Autodesk Inventor part; units mm, degrees
ref_plane "YZ Plane" through (0, 0, 0) normal (1, 0, 0) x (0, 1, 0)
ref_plane "XZ Plane" through (0, 0, 0) normal (0, 1, 0) x (-1, 0, 0)
ref_plane "XY Plane" through (0, 0, 0) normal (0, 0, 1) x (1, 0, 0)
sketch "Sketch1" plane through (0, 0, 0) normal (0, 1, 0) x (-1, 0, 0)
  line L0 (95, 92.5) -> (-95, 92.5)
  line L1 (-95, 92.5) -> (-95, -92.5)
  line L2 (-95, -92.5) -> (95, -92.5)
  line L3 (95, -92.5) -> (95, 92.5)
  point P0 (0, 0)
  dimension "d0" = 190
  dimension "d1" = 185
  dimension "d2" = 92.5
  dimension "d3" = 95
extrude "Extrusion1" add sketch "Sketch1" against normal blind 15
sketch "Sketch5" plane through (0, 0, 0) normal (0, 1, 0) x (1, 0, 0)
  line L0 (-95, -92.5) -> (95, -92.5)
  line L1 (95, -92.5) -> (95, 92.5)
  line L2 (95, 92.5) -> (-95, 92.5)
  line L3 (-95, 92.5) -> (-95, -92.5)
  line L4 (-89.5, -87) -> (89.5, -87)
  line L5 (89.5, -87) -> (89.5, 87)
  line L6 (89.5, 87) -> (-89.5, 87)
  line L7 (-89.5, 87) -> (-89.5, -87)
  point P0 (0, 0)
  dimension "d42" = 5.5
  dimension "d43" = 5.5
  dimension "d44" = 5.5
  dimension "d45" = 5.5
extrude "Extrusion6" add sketch "Sketch5" along normal blind 14 contours L7 L6 L5 L4
sketch "Sketch6" plane through (0, 14, 0) normal (0, 1, 0) x (1, 0, 0)
  line L0 (-89.5, -87) -> (89.5, -87)
  line L1 (89.5, -87) -> (89.5, 87)
  line L2 (89.5, 87) -> (-89.5, 87)
  line L3 (-89.5, 87) -> (-89.5, -87)
  line L4 (87, -84.5) -> (-87, -84.5)
  line L5 (-87, -84.5) -> (-87, 84.5)
  line L6 (-87, 84.5) -> (87, 84.5)
  line L7 (87, 84.5) -> (87, -84.5)
  point P0 (0, 0)
  dimension "d48" = 2.5
  dimension "d49" = 2.5
  dimension "d50" = 2.5
  dimension "d51" = 2.5
extrude "Extrusion7" cut sketch "Sketch6" against normal blind 15 contours L4 L5 L6 L7
sketch "Sketch7" plane through (0, -15, 0) normal (0, -1, 0) x (1, 0, 0)
  line L0 (95, 92.5) -> (-95, 92.5)
  line L1 (-95, 92.5) -> (-95, -92.5)
  line L2 (-95, -92.5) -> (95, -92.5)
  line L3 (95, -92.5) -> (95, 92.5)
  line L4 (90, 87.5) -> (-90, 87.5)
  line L5 (-90, 87.5) -> (-90, -87.5)
  line L6 (-90, -87.5) -> (90, -87.5)
  line L7 (90, -87.5) -> (90, 87.5)
  point P0 (0, 0)
  dimension "d54" = 5
  dimension "d55" = 5
  dimension "d56" = 5
  dimension "d57" = 5
extrude "Extrusion8" cut sketch "Sketch7" against normal blind 10 contours L7 L6 L5 L4
sketch "Sketch8" plane through (0, -1, 0) normal (0, 1, 0) x (1, 0, 0)
  line L0 (87, -84.5) -> (-87, -84.5)
  line L1 (87, 84.5) -> (87, -84.5)
  line L2 (-87, 84.5) -> (87, 84.5)
  line L3 (-87, -84.5) -> (-87, 84.5)
  line L4 (-67, -64.5) -> (67, -64.5)
  line L5 (67, -64.5) -> (67, 64.5)
  line L6 (67, 64.5) -> (-67, 64.5)
  line L7 (-67, 64.5) -> (-67, -64.5)
  line L8 (-57, -54.5) -> (57, -54.5)
  line L9 (57, -54.5) -> (57, 54.5)
  line L10 (57, 54.5) -> (-57, 54.5)
  line L11 (-57, 54.5) -> (-57, -54.5)
  line L12 (-67, -44.5) -> (-57, -44.5)
  line L13 (-47, -64.5) -> (-47, -54.5)
  line L14 (-67, 44.5) -> (-57, 44.5)
  line L15 (-47, 54.5) -> (-47, 64.5)
  line L16 (47, -64.5) -> (47, -54.5)
  line L17 (57, -44.5) -> (67, -44.5)
  line L18 (47, 54.5) -> (47, 64.5)
  line L19 (57, 44.5) -> (67, 44.5)
  point P0 (0, 0)
  dimension "d60" = 20
  dimension "d61" = 20
  dimension "d62" = 20
  dimension "d63" = 20
  dimension "d64" = 10
  dimension "d65" = 10
  dimension "d66" = 10
  dimension "d67" = 10
  dimension "d68" = 20
  dimension "d69" = 20
  dimension "d70" = 20
  dimension "d71" = 20
  dimension "d72" = 20
  dimension "d73" = 20
  dimension "d74" = 20
  dimension "d75" = 20
extrude "Extrusion9" cut sketch "Sketch8" against normal through all contours L13 L8 L16 L4 | L17 L9 L19 L5 | L6 L18 L10 L15
sketch "Sketch9" plane through (0, -1, 0) normal (0, 1, 0) x (1, 0, 0)
  line L0 (47, -54.5) -> (47, -64.5)
  line L1 (47, -64.5) -> (-47, -64.5)
  line L2 (-47, -64.5) -> (-47, -54.5)
  line L3 (-47, -54.5) -> (47, -54.5)
  line L4 (67, 44.5) -> (67, -44.5)
  line L5 (67, -44.5) -> (57, -44.5)
  line L6 (57, -44.5) -> (57, 44.5)
  line L7 (57, 44.5) -> (67, 44.5)
  line L8 (47, 64.5) -> (47, 54.5)
  line L9 (47, 54.5) -> (-47, 54.5)
  line L10 (-47, 54.5) -> (-47, 64.5)
  line L11 (-47, 64.5) -> (47, 64.5)
  line L12 (87, -84.5) -> (-87, -84.5)
  line L13 (87, 84.5) -> (87, -84.5)
  line L14 (-87, 84.5) -> (87, 84.5)
  line L15 (-87, -84.5) -> (-87, 84.5)
  line L16 (-75, -10) -> (-20, -10)
  line L17 (-20, -10) -> (-20, 10)
  line L18 (-20, 10) -> (-75, 10)
  line L19 (-75, 10) -> (-75, -10)
  point P0 (0, 0)
  dimension "d78" = 55
  dimension "d79" = 20
  dimension "d80" = 20
  dimension "d81" = 10
extrude "Extrusion10" cut sketch "Sketch9" against normal through all contours L19 L18 L17 L16
equation "\"d43\" = d42"
equation "\"d44\" = d42"
equation "\"d45\" = d42"
equation "\"d49\" = d48"
equation "\"d50\" = d48"
equation "\"d51\" = d48"
equation "\"d55\" = d54"
equation "\"d56\" = d54"
equation "\"d57\" = d54"
equation "\"d61\" = d60"
equation "\"d62\" = d60"
equation "\"d63\" = d60"
equation "\"d65\" = d64"
equation "\"d66\" = d64"
equation "\"d67\" = d64"
equation "\"d68\" = d69"
equation "\"d70\" = d69"
equation "\"d71\" = d69"
equation "\"d72\" = d69"
equation "\"d73\" = d69"
equation "\"d74\" = d69"
equation "\"d75\" = d69"
properties part number "Platform"
Could you check a few things on this model? Use its own coordinates, in mm. A direction names the side the tool comes from. Give positions to 0.01 mm unless a question says otherwise; leave off trailing zeros. Order: outer loops, then holes, each group sorted by start corner. A loop starts at its lowest first (then second) coordinate and runs counter-clockwise, first axis right, second up.
1. Suppose I cut it at C-C (y = 5.5). Write out the boundary of the cut face in (x, z).
Answers below:
outline: (-89.5, -87) - (89.5, -87) - (89.5, 87) - (-89.5, 87) - close; hole (-87, -84.5) - (87, -84.5) - (87, 84.5) - (-87, 84.5) - close
2. Suppose I cut it at D-D (x = 11.5). Write out the boundary of the cut face in (y, z), plus the area to 3 significant figures.
Answers below:
outline: (-15, -92.5) - (0, -92.5) - (0, -87) - (14, -87) - (14, -84.5) - (-1, -84.5) - (-1, -64.5) - (-5, -64.5) - (-5, -87.5) - (-15, -87.5) - close; (-15, 87.5) - (-5, 87.5) - (-5, 64.5) - (-1, 64.5) - (-1, 84.5) - (14, 84.5) - (14, 87) - (0, 87) - (0, 92.5) - (-15, 92.5) - close; (-5, -54.5) - (-1, -54.5) - (-1, 54.5) - (-5, 54.5) - close
area: 846 mm2
3. Which directions (+Z, -Z, +X, -X, +Y, -Y) give clear straight access to the entire face, cutting with the end or side of a thin tool? Please do faces 4 (the flat face through (1, 7, -87)), 5 (the flat face through (-1, 7, 87)), 6 (the flat face through (90, -10, -1)).
Answers below:
face 4: -Z, +X, -X, +Y
face 5: +Z, +X, -X, +Y
face 6: -Y
4. Suppose I cut it at A-A (z = -20). Write out the boundary of the cut face in (x, y), plus the area to 3 significant figures.
Answers below:
outline: (-95, -15) - (-90, -15) - (-90, -5) - (57, -5) - (57, -1) - (-87, -1) - (-87, 14) - (-89.5, 14) - (-89.5, 0) - (-95, 0) - close; (67, -5) - (90, -5) - (90, -15) - (95, -15) - (95, 0) - (89.5, 0) - (89.5, 14) - (87, 14) - (87, -1) - (67, -1) - close
area: 906 mm2
5. For pin 1 (4 mm diameter, centred on y = 1.5, z = 35, fed in from -X); pin 2 (2 mm diameter, centred on x = 36, z = 7, fed in from +Y); pin 3 (7.5 mm diameter, centred on x = -1, y = 9.5, fed in from +Z); pin 4 (11 mm diameter, centred on x = -27, y = 6.5, fed in from -Z), each with a flat end and sliding along its axis, tell me the tip position at first contact or that it passes through.
Answers below:
pin 1: stops at x = -95
pin 2: stops at y = -1
pin 3: stops at z = 87
pin 4: stops at z = -87
6. Suppose I cut it at B-B (x = -64). Write out the boundary of the cut face in (y, z), plus the area to 3 significant figures.
Answers below:
outline: (-15, -92.5) - (0, -92.5) - (0, -87) - (14, -87) - (14, -84.5) - (-1, -84.5) - (-1, -10) - (-5, -10) - (-5, -87.5) - (-15, -87.5) - close; (-15, 87.5) - (-5, 87.5) - (-5, 10) - (-1, 10) - (-1, 84.5) - (14, 84.5) - (14, 87) - (0, 87) - (0, 92.5) - (-15, 92.5) - close
area: 846 mm2
7. I need wall thicknesses on L1, parallel to Z at x = -8, y = -2.75; L2, parallel to X at y = 8.5, z = -82; L3, parallel to X at y = -7.75, z = -54.5. Which ranges of each line are inside material? Lowest first, please.
Answers below:
L1: z = -92.5 to -64.5, -54.5 to 54.5, 64.5 to 92.5
L2: x = -89.5 to -87, 87 to 89.5
L3: x = -95 to -90, 90 to 95
8. Thinking about a two-plate mould opening in X: for faces 1 (the flat face through (1, -10, 87.5)), 2 (the flat face through (89.5, 7, 1)), 3 (the flat face through (7, 0, -89)), which applies, +X half, -X half, draft (parallel to the pull), parting line (faces both ways), or undercut?
Answers below:
face 1: undercut
face 2: +X half
face 3: draft
